Check sheet for the modelled part. Datum: model origin and axes. Units: mm. Give positions to 0.01 mm unless a question says otherwise; leave off trailing zeros. One line per question, with ' | ' between items.
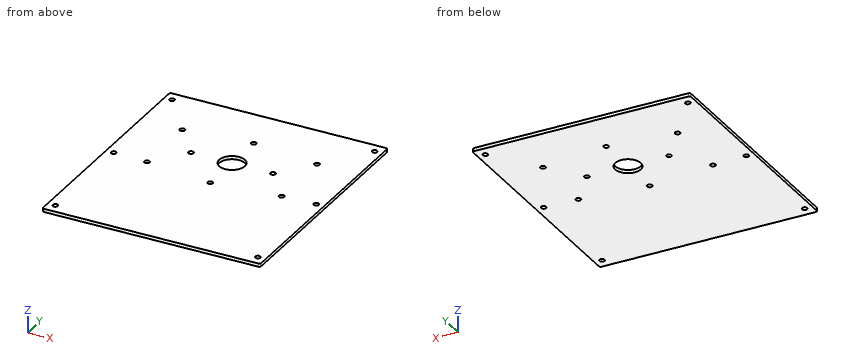
```python
from build123d import *

# Parameters (mm, degrees)
SKETCH1_R           = 20
SKETCH1_R_2         = 4
BOSS_EXTRUDE1_DEPTH = 5


with BuildPart() as part:
    # Sketch1 → Boss-Extrude1 (new body)
    with BuildSketch(Plane.XY.offset(5)):
        with BuildLine():
            Line((-170, 184.5), (-170, -184.5))
            ThreePointArc((-170, -184.5), (-169.121320344, -186.621320344), (-167, -187.5))
            Line((-167, -187.5), (167, -187.5))
            ThreePointArc((167, -187.5), (169.121320344, -186.621320344), (170, -184.5))
            Line((170, -184.5), (170, 184.5))
            ThreePointArc((170, 184.5), (169.121320344, 186.621320344), (167, 187.5))
            Line((167, 187.5), (-167, 187.5))
            ThreePointArc((-167, 187.5), (-169.121320344, 186.621320344), (-170, 184.5))
        make_face()
        with Locations((0, 50)):
            Circle(SKETCH1_R, mode=Mode.SUBTRACT)
        with Locations((-64, 50)):
            Circle(SKETCH1_R_2, mode=Mode.SUBTRACT)
        with Locations((0, 114)):
            Circle(SKETCH1_R_2, mode=Mode.SUBTRACT)
        with Locations((64, 50)):
            Circle(SKETCH1_R_2, mode=Mode.SUBTRACT)
        with Locations((0, -14)):
            Circle(SKETCH1_R_2, mode=Mode.SUBTRACT)
        with Locations((158, 0)):
            Circle(SKETCH1_R_2, mode=Mode.SUBTRACT)
        with Locations((-158, 0)):
            Circle(SKETCH1_R_2, mode=Mode.SUBTRACT)
        with Locations((158, 171.5)):
            Circle(SKETCH1_R_2, mode=Mode.SUBTRACT)
        with Locations((-158, 171.5)):
            Circle(SKETCH1_R_2, mode=Mode.SUBTRACT)
        with Locations((-158, -171.5)):
            Circle(SKETCH1_R_2, mode=Mode.SUBTRACT)
        with Locations((158, -171.5)):
            Circle(SKETCH1_R_2, mode=Mode.SUBTRACT)
        with Locations((-105, 102)):
            Circle(SKETCH1_R_2, mode=Mode.SUBTRACT)
        with Locations((-105, -2)):
            Circle(SKETCH1_R_2, mode=Mode.SUBTRACT)
        with Locations((105, 102)):
            Circle(SKETCH1_R_2, mode=Mode.SUBTRACT)
        with Locations((105, -2)):
            Circle(SKETCH1_R_2, mode=Mode.SUBTRACT)
    extrude(amount=-BOSS_EXTRUDE1_DEPTH)


solid = part.part
```
Q1. Depth check by flat-ended pin: pin 1 Ø13 at (x, y) = (-64, 50) entering from +Z. Enter the tip coordinate at first touch or a pass-through.
Result sheet:
pin 1: stops at z = 5
Q2. Thickness scan on line 1 (X direction, y = -172, z = 3.75); line 2 (Y direction, x = 158, z = 1.2); line 3 (Y direction, x = 0, z = 2.9). Record the ranges inside material, lowest first.
Result sheet:
line 1: x = -170 to -161.97, -154.03 to 154.03, 161.97 to 170 | line 2: y = -187.5 to -175.5, -167.5 to -4, 4 to 167.5, 175.5 to 187.5 | line 3: y = -187.5 to -18, -10 to 30, 70 to 110, 118 to 187.5
Q3. Section check A-A (z = 2.45). Count the separate pieces of the cut face and the enclosed holes in it, and give its area (3 significant figures).
Result sheet:
separate pieces: 1 | enclosed holes: 15 | area: 126,000 mm2
